from build123d import *

# Parameters (mm, degrees)
SKETCH_1_W           = 21.6
SKETCH_1_H           = 25
EXTRUDE_1_DEPTH      = 10
SKETCH_2_W           = 44
SKETCH_2_H           = 36
EXTRUDE_2_DEPTH      = 3
EXTRUDE_3_DEPTH      = 2
EXTRUDE_3_DEPTH_BACK = 23.6
SKETCH_3_W           = 6
SKETCH_3_H           = 25
CHAMFER_1_SIZE       = 1
SKETCH_4_W           = 16
SKETCH_4_H           = 25
CUT_EXTRUDE_1_DEPTH  = 10
FILLET_1_R           = 2
SKETCH_5_W           = 15.991126726
SKETCH_5_H           = 26
CUT_EXTRUDE_2_DEPTH  = 34.708307581
FILLET_2_R           = 2
FILLET_START         = 5.4999999
FILLET_3_DEPTH       = 7.0000001
FILLET_START_2       = -12.5
FILLET_3_2_DEPTH     = 18.304364073
FILLET_START_3       = 8
FILLET_3_3_DEPTH     = 2


with BuildPart() as part:
    # ｽｹｯﾁ1 → ﾎﾞｽ - 押し出し1 (new body)
    with BuildSketch(Plane.XY):
        Rectangle(SKETCH_1_W, SKETCH_1_H)
    extrude(amount=EXTRUDE_1_DEPTH)

    # ｽｹｯﾁ2 → ﾎﾞｽ - 押し出し2 (add)
    with BuildSketch(Plane.XY.offset(10)):
        with Locations((0, -5.5)):
            Rectangle(SKETCH_2_W, SKETCH_2_H)
    extrude(amount=EXTRUDE_2_DEPTH)

    # ｽｹｯﾁ3 → ﾎﾞｽ - 押し出し3 (add, two sides: drawn at the far end of the back side and taken through both)
    with BuildSketch(Plane(origin=(10.8, 0, 0), x_dir=(0, 0, -1), z_dir=(1, 0, 0)).offset(-EXTRUDE_3_DEPTH_BACK)):
        with Locations((-7, 0)):
            Rectangle(SKETCH_3_W, SKETCH_3_H)
    extrude(amount=EXTRUDE_3_DEPTH + EXTRUDE_3_DEPTH_BACK)

    # 面取り1
    chamfer_1_edges = [part.edges().sort_by_distance(p)[0] for p in [
        (-10.8, 0, 0),
        (10.8, 0, 0),
    ]]
    chamfer(chamfer_1_edges, length=CHAMFER_1_SIZE)

    # ｽｹｯﾁ4 → ｶｯﾄ - 押し出し1 (cut)
    with BuildSketch(Plane(origin=(0, 0, 0), x_dir=(-1, 0, 0), z_dir=(0, 0, -1))):
        Rectangle(SKETCH_4_W, SKETCH_4_H)
    extrude(amount=-CUT_EXTRUDE_1_DEPTH, mode=Mode.SUBTRACT)

    # ﾌｨﾚｯﾄ1
    fillet_1_edges = [part.edges().sort_by_distance(p)[0] for p in [
        (22, -23.5, 11.5),
        (22, 12.5, 11.5),
        (-22, 12.5, 11.5),
        (-22, -23.5, 11.5),
    ]]
    fillet(fillet_1_edges, radius=FILLET_1_R)

    # ｽｹｯﾁ5 → ｶｯﾄ - 押し出し2 (cut, through all)
    with BuildSketch(Plane(origin=(0, 0, 10), x_dir=(-1, 0, 0), z_dir=(0, 0, -1))):
        with Locations((0, -5.5)):
            Rectangle(SKETCH_5_W, SKETCH_5_H)
    extrude(amount=-CUT_EXTRUDE_2_DEPTH, mode=Mode.SUBTRACT)

    # ﾌｨﾚｯﾄ2
    fillet_2_edges = [part.edges().sort_by_distance(p)[0] for p in [
        (-7.995563363, 7.5, 11.5),
        (-7.995563363, -18.5, 11.5),
        (7.995563363, -18.5, 11.5),
        (7.995563363, 7.5, 11.5),
    ]]
    fillet(fillet_2_edges, radius=FILLET_2_R)

    # ﾌｨﾚｯﾄ3: read off the stored shape, not the designer's step
    # ﾌｨﾚｯﾄ3 outline → ﾌｨﾚｯﾄ3 (add)
    with BuildSketch(Plane(origin=(0, 0, 0), x_dir=(1, 0, 0), z_dir=(0, 1, 0)).offset(FILLET_START)):
        with BuildLine():
            ThreePointArc((-6, -10), (-7.414213562, -9.414213562), (-8, -8))
            Line((-8, -8), (-8, -10))
            Line((-8, -10), (-6, -10))
        make_face()
        with BuildLine():
            Line((6, -10), (8, -10))
            Line((8, -10), (8, -8))
            ThreePointArc((8, -8), (7.414213562, -9.414213562), (6, -10))
        make_face()
    extrude(amount=FILLET_3_DEPTH)

    # Fillet 3 2 outline → Fillet 3 2 (add)
    with BuildSketch(Plane(origin=(0, 0, 0), x_dir=(1, 0, 0), z_dir=(0, 1, 0)).offset(FILLET_START_2)):
        with BuildLine():
            Line((-7.995563363, -10), (-7.995563363, -8.133142264))
            ThreePointArc((-7.995563363, -8.133142264), (-7.998890533, -8.066608082), (-8, -8))
            Line((-8, -8), (-8, -10))
            Line((-8, -10), (-7.995563363, -10))
        make_face()
        with BuildLine():
            ThreePointArc((8, -8), (7.998890533, -8.066608082), (7.995563363, -8.133142264))
            Line((7.995563363, -8.133142264), (7.995563363, -10))
            Line((7.995563363, -10), (8, -10))
            Line((8, -10), (8, -8))
        make_face()
    extrude(amount=FILLET_3_2_DEPTH)

    # Fillet 3 3 outline → Fillet 3 3 (cut)
    with BuildSketch(Plane.XY.offset(FILLET_START_3)):
        with BuildLine():
            Line((5.995563363, 7.5), (-5.995563363, 7.5))
            ThreePointArc((-5.995563363, 7.5), (-7.409776925, 6.914213563), (-7.995563363, 5.5))
            Line((-7.995563363, 5.5), (7.995563363, 5.5))
            ThreePointArc((7.995563363, 5.5), (7.409776925, 6.914213563), (5.995563363, 7.5))
        make_face()
    extrude(amount=FILLET_3_3_DEPTH, mode=Mode.SUBTRACT)


solid = part.part
For this review, take the finished solid that the model builds, in its own axes (mm). A direction names the side the tool comes from. Round coordinates to 2 decimals unless told otherwise and drop trailing zeros. Loops run counter-clockwise (first coordinate to the right, second up) from the corner with the lowest first, then second, coordinate; pieces in that order, holes last. Notation, with made-up numbers: (-6.75, 78.5) - (0.25, 78.5) arc R11 ccw to (0.25, 96.5) - close; hole circle Ø6 at (4.25, 2.25). An arc over 180 degrees is marked (long way). Use one line per item in the form item = value.
Item 1: Consider section A-A on z = 3.5. Write out the cut boundary in (x, y).
Answers:
outline = (-10.8, -12.5) - (-8, -12.5) - (-8, 12.5) - (-10.8, 12.5) - close; (8, -12.5) - (10.8, -12.5) - (10.8, 12.5) - (8, 12.5) - close
Item 2: Consider section B-B on x = 4. Write out the cut boundary in (y, z), then the cut area to 3 significant figures.
Answers:
outline = (-23.5, 10) - (-18.5, 10) - (-18.5, 13) - (-23.5, 13) - close; (7.5, 10) - (12.5, 10) - (12.5, 13) - (7.5, 13) - close
area = 30.0 mm^2
Item 3: Consider section C-C on y = -9. Write out the cut boundary in (x, z).
Answers:
outline = (-22, 10) - (-12.8, 10) - (-12.8, 4) - (-10.8, 4) - (-10.8, 1) - (-9.8, 0) - (-8, 0) - (-8, 8) arc R2 cw to (-8, 8.13) - (-8, 13) - (-22, 13) - close; (8, 0) - (9.8, 0) - (10.8, 1) - (10.8, 4) - (12.8, 4) - (12.8, 10) - (22, 10) - (22, 13) - (8, 13) - (8, 8.13) arc R2 cw to (8, 8) - close
Item 4: Tool access review of faces 1 (the flat face through (-10.8, 0, 2)), 2 (the flat face through (0, 7.5, 11)), 3 (the flat face through (12.8, 0, 7)), 4 (the flat face through (8, 0, 4)), 5 (the flat face through (-10, -12.5, 6)): name each direction out of +Z, -Z, +X, -X, +Y, -Y from which nothing blocks a thin tool from reaching the whole face with its end or side.
Answers:
face_1 = -Z, -X, +Y, -Y
face_2 = +Z, -Z
face_3 = -Z, +X, +Y, -Y
face_4 = -Z, +Y, -Y
face_5 = -Z, +X, -X, -Y
Item 5: Clearance check with flat-ended pins moving along their axes: P1, Ø1.5, axis at x = 11.5, z = 3, coming from the -Y side; P2, Ø6.5, axis at y = 5.5, z = 3, coming from the -X side; P3, Ø1.6, axis at x = 12, y = 4.5, coming from the -Z side. State where each tip first meets the part, or that it passes through.
Answers:
P1 = -12.5
P2 = -12.8
P3 = 4
Item 6: Mouldability with a two-part tool opening along Y and no side actions: class faces 6 (the cylindrical face through (-21.43, -22.9, 11.52)), 7 (the flat face through (12, 0, 4)), 8 (the cylindrical face through (-7.425, -17.899, 11.521)) as +Y half, -Y half, draft (parallel to the pull), parting line (faces both ways), or undercut.
Answers:
face_6 = -Y half
face_7 = draft
face_8 = undercut
Item 7: For line 1 (X direction, y = 11.5, z = 8); line 2 (X direction, y = -8.5, z = 3); line 3 (Z direction, x = 11.5, y = 0.5), list the stretches that pass through material, from the lowest coordinate up.
Answers:
line_1 = -12.8 to -8, 8 to 12.8
line_2 = -10.8 to -8, 8 to 10.8
line_3 = 4 to 13
Item 8: Consider section D-D on z = 12. Write out the cut boundary in (x, y), then the cut area to 3 significant figures.
Answers:
outline = (-22, -21.5) arc R2 ccw to (-20, -23.5) - (20, -23.5) arc R2 ccw to (22, -21.5) - (22, 10.5) arc R2 ccw to (20, 12.5) - (-20, 12.5) arc R2 ccw to (-22, 10.5) - close; hole (-8, -16.5) arc R2 ccw to (-6, -18.5) - (6, -18.5) arc R2 ccw to (8, -16.5) - (8, 5.5) arc R2 ccw to (6, 7.5) - (-6, 7.5) arc R2 ccw to (-8, 5.5) - close
area = 1,170 mm^2
